Geometry check sheet. Reference: the model listing, model coordinates, mm. Coordinates: 2 decimals unless noted, no trailing zeros. Write each loop counter-clockwise with the first axis right and the second up, starting at its lowest first coordinate (ties: lowest second). Pieces come first, ordered by that corner, then holes. Notation, with made-up numbers: (-4.75, 50.5) - (20.25, 50.5) arc R13 ccw to (20.25, 71.5) - close; hole circle Ø4 at (59, 29.25). An arc over 180 degrees is marked (long way). Answer as a JSON object with one key per item and string values. Group by question number.
from build123d import *

# Parameters (mm, degrees)
SKETCH_1_W          = 50
SKETCH_1_H          = 100
EXTRUDE_1_DEPTH     = 10
SKETCH_2_R          = 4
CUT_EXTRUDE_1_DEPTH = 113.249721603
CHAMFER_1_SIZE      = 6


with BuildPart() as part:
    # 草图1 → 凸台-拉伸1 (new, symmetric)
    with BuildSketch(Plane.XY):
        with Locations((0, 50)):
            Rectangle(SKETCH_1_W, SKETCH_1_H)
    extrude(amount=EXTRUDE_1_DEPTH, both=True)

    # 草图2 → 切除-拉伸1 (cut, through all)
    with BuildSketch(Plane.ZY.offset(25)):
        with Locations((0, 7.522576351)):
            Circle(SKETCH_2_R)
    extrude(amount=-CUT_EXTRUDE_1_DEPTH, mode=Mode.SUBTRACT)

    # 倒角1
    chamfer_1_edges = [part.edges().sort_by_distance(p)[0] for p in [
        (0, 0, 10),
        (0, 0, -10),
    ]]
    chamfer(chamfer_1_edges, length=CHAMFER_1_SIZE)


solid = part.part
(1) Section check C-C (z = -7). Record the cut outline in (x, y).
(2) Section check A-A (z = 0). Record the cut outline in (x, y).
(3) Section check B-B (x = 14). Record the cut outline in (y, z), and give its area (3 significant figures).
(4) Gauge pin test, flat end, axial feed: pin 1 (2 mm diameter, centred on x = -10.5, z = -7.5, fed in from -Y). Record the tip position at first contact, or that the pin passes through.
(5) Draft check along Y on faces 1 (the face through (-0.35, 3.62, -0.87)), 2 (the face through (0, 100, 0)), 3 (the face through (0, 3, -7)). Enter one of: +Y half, -Y half, draft (parallel to the pull), parting line (faces both ways), or undercut.
(6) Material ranges on L1, parallel to Y at x = -7, z = 0; L2, parallel to Y at x = -11, z = -2.25; L3, parallel to Y at x = -16.5, z = -9, recorded low to high. Write a range as [from, to].
Conclusion:
{
 "1": {"outline": "(-25, 3) - (25, 3) - (25, 100) - (-25, 100) - close"},
 "2": {"outline": "(-25, 0) - (25, 0) - (25, 3.52) - (-25, 3.52) - close; (-25, 11.52) - (25, 11.52) - (25, 100) - (-25, 100) - close"},
 "3": {"outline": "(0, -4) - (6, -10) - (100, -10) - (100, 10) - (6, 10) - (0, 4) - close; hole circle Ø8 at (7.52, 0)", "area": "1,910 mm^2"},
 "4": {"pin 1": "stops at y = 2.5"},
 "5": {"face 1": "undercut", "face 2": "+Y half", "face 3": "-Y half"},
 "6": {"L1": "y = [0, 3.52], [11.52, 100]", "L2": "y = [0, 4.22], [10.83, 100]", "L3": "y = [5, 100]"}
}
